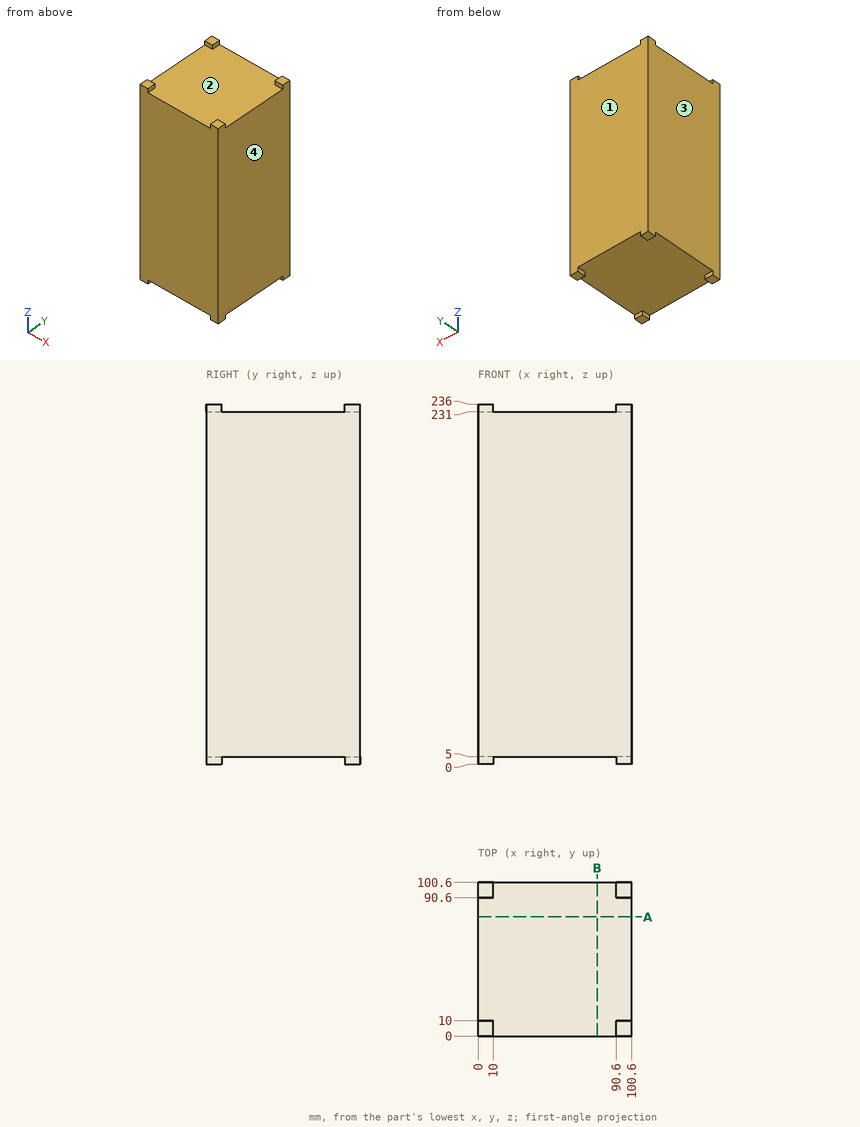
Geometry check sheet. Reference: drawing and pictorial views, mm from the part's lowest x, y, z. Round coordinates to 2 decimals unless told otherwise and drop trailing zeros. Loops run counter-clockwise (first coordinate to the right, second up) from the corner with the lowest first, then second, coordinate; pieces in that order, holes last.
1. Gauge pin test, flat ends, axial feed: pin 1 Ø5 at (x, y) = (28.5, 17.5) entering from -Z; pin 2 Ø6 at (x, y) = (19, 29.5) entering from +Z. Record the tip position at first contact, or that the pin passes through.
2. Mould release check, pull along X, two halves, no side actions. Record for the marked faces 1, 2, 3 and 4: released by +X, released by -X, zero draft, split by the parting line, or undercut.
3. Scan line: probe 1 along Z at (x, y) = (43, 79.5). Record every from-to range of solid material in increasing order.
4. Sectioned sample at A-A on y = 78. Record the boundary of the cut face in (x, z).
Recorded:
1. pin 1: stops at z = 5
1. pin 2: stops at z = 231
2. face 1: zero draft
2. face 2: undercut
2. face 3: released by -X
2. face 4: released by +X
3. probe 1: z = 5 to 231
4. outline: (0, 5) - (100.6, 5) - (100.6, 231) - (0, 231) - close
